Could you check a few things on this drawing? It's one solid part, dimensions in mm from its lowest x, y, z. A direction names the side the tool comes from. Give positions to 0.01 mm unless a question says otherwise; leave off trailing zeros. Order: outer loops, then holes, each group sorted by start corner. A loop starts at its lowest first (then second) coordinate and runs counter-clockwise, first axis right, second up. Notation, with made-up numbers: (12, 89.5) - (70, 89.5) arc R12 ccw to (70, 96.5) - close; hole circle Ø3 at (-23.5, -9.75). An arc over 180 degrees is marked (long way). Answer as CSV lines item,"result".
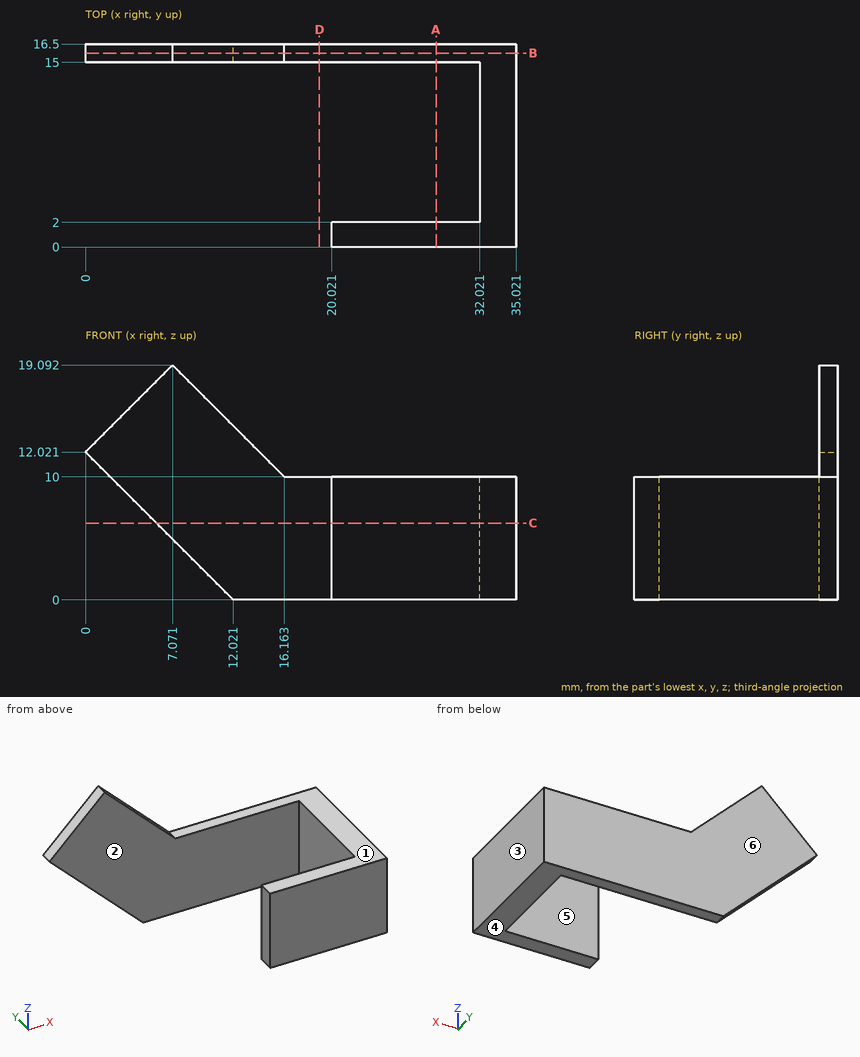
1) I'm going to push flat-ended pins straight in: P1, Ø0.6, axis at y = 1, z = 5, coming from the -X side; P2, Ø10, axis at x = 9.5, z = 3, coming from the -Y side; P3, Ø5.5, axis at x = 21.5, z = 9, coming from the -Y side. Where does each tip first touch, or does it pass through?
Answer block:
P1,"x = 20.02"
P2,"y = 15"
P3,"y = 0"
2) I want a section at A-A on x = 28.5. Write out the boundary of the cut face in (y, z), plus the area to 3 significant figures.
Answer block:
outline,"(0, 0) - (2, 0) - (2, 10) - (0, 10) - close; (15, 0) - (16.5, 0) - (16.5, 10) - (15, 10) - close"
area,"35.0 mm2"
3) I want a section at C-C on z = 6.25. Write out the boundary of the cut face in (x, y).
Answer block:
outline,"(5.77, 15) - (32.02, 15) - (32.02, 2) - (20.02, 2) - (20.02, 0) - (35.02, 0) - (35.02, 16.5) - (5.77, 16.5) - close"
4) I want a section at D-D on x = 19. Write out the boundary of the cut face in (y, z), plus the area to 3 significant figures.
Answer block:
outline,"(15, 0) - (16.5, 0) - (16.5, 10) - (15, 10) - close"
area,"15.0 mm2"
5) Which directions (+Z, -Z, +X, -X, +Y, -Y) give clear straight access to the entire face, cutting with the end or side of a thin tool? Please do the marked faces 1, 2 and 3.
Answer block:
face 1,"+Z, +X, +Y, -Y"
face 2,"+Z, -Z, -X"
face 3,"+Z, -Z, +X, +Y, -Y"
6) I want a section at B-B on y = 15.75. Write out the boundary of the cut face in (x, z).
Answer block:
outline,"(0, 12.02) - (12.02, 0) - (35.02, 0) - (35.02, 10) - (16.16, 10) - (7.07, 19.09) - close"
7) If we mould it in two halves opening along Y, with no side actions, what happens to the marked faces 4, 5 and 6? For each: +Y half, -Y half, draft (parallel to the pull), parting line (faces both ways), or undercut.
Answer block:
face 4,"draft"
face 5,"undercut"
face 6,"+Y half"
8) I need wall thicknesses on line 1 along Y through (x, z) = (20.5, 8.25); line 2 along Y through (x, z) = (13, 11.75); line 3 along X through (y, z) = (9.5, 5.5). Which ranges of each line are inside material? Lowest first, please. Write a range as [from, to].
Answer block:
line 1,"[0, 2], [15, 16.5]"
line 2,"[15, 16.5]"
line 3,"[32.02, 35.02]"
